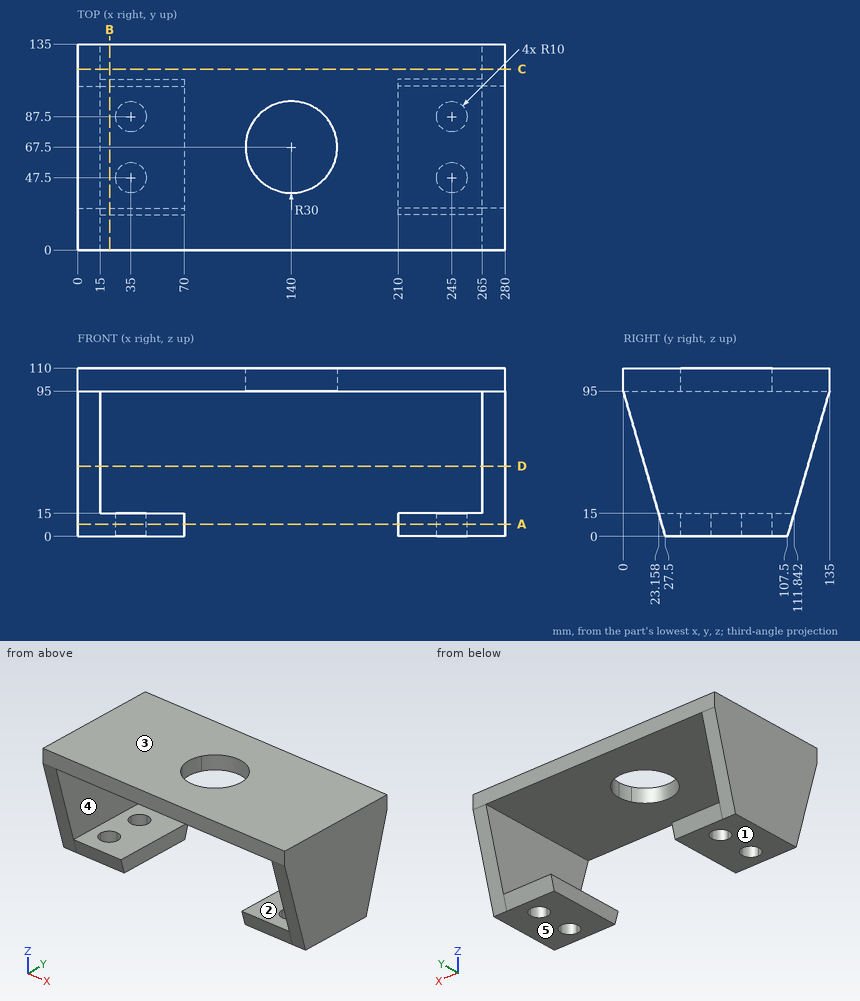
Can you work these out from the drawing? Everything is in mm from the part's minimum corner. A direction names the side the tool comes from. Round coordinates to 2 decimals unless told otherwise and drop trailing zeros. Write each loop counter-clockwise with the first axis right and the second up, starting at its lowest first coordinate (ties: lowest second). Pieces come first, ordered by that corner, then holes. Notation, with made-up numbers: (33.25, 79) - (48.25, 79) arc R21 cw to (48.25, 112) - close; hole circle Ø3 at (74.25, -0.5). An arc over 180 degrees is marked (long way). Write each question's results on one line, items separated by ' | '. Start each with the question number.
1) Please list where these lines run through material, in increasing order: line 1 (Z direction, x = 223, y = 82.5); line 2 (X direction, y = 30, z = 62.5); line 3 (Z direction, x = 82, y = 76.5).
2) Which directions (+Z, -Z, +X, -X, +Y, -Y) give clear straight access to the entire face, cutting with the end or side of a thin tool? Please do the marked faces 1 and 2.
3) Suppose I cut it at B-B (x = 21). List the corners of the cut face in (y, z) for me, and give its area (3 significant figures).
4) We'd pull the mould along Z, two halves only. Please class the marked faces 3, 4 and 5: released by +Z, released by -Z, zero draft, split by the parting line, or undercut.
5) Suppose I cut it at C-C (y = 118.5). List the corners of the cut face in (x, z) for me.
6) Suppose I cut it at D-D (z = 46). List the corners of the cut face in (x, y) for me.
7) Suppose I cut it at A-A (z = 8). List the corners of the cut face in (x, y) for me, and give its area (3 significant figures).
8) For pin 1 Ø6 at (x, z) = (216.5, 18.5) entering from -Y, with a flat end and sliding along its axis, tell me the tip position at first contact or that it passes through.
Here are the results:
1) line 1: z = 0 to 15, 95 to 110 | line 2: x = 0 to 15, 265 to 280 | line 3: z = 95 to 110
2) face 1: -Z, +X, -X, +Y, -Y | face 2: +Y, -Y
3) outline: (0, 95) - (135, 95) - (135, 110) - (0, 110) - close; (23.16, 15) - (27.5, 0) - (107.5, 0) - (111.84, 15) - close | area: 3,290 mm2
4) face 3: released by +Z | face 4: undercut | face 5: released by -Z
5) outline: (0, 38) - (15, 38) - (15, 95) - (265, 95) - (265, 38) - (280, 38) - (280, 110) - (0, 110) - close
6) outline: (0, 14.18) - (15, 14.18) - (15, 120.82) - (0, 120.82) - close; (265, 14.18) - (280, 14.18) - (280, 120.82) - (265, 120.82) - close
7) outline: (0, 25.18) - (70, 25.18) - (70, 109.82) - (0, 109.82) - close; (210, 25.18) - (280, 25.18) - (280, 109.82) - (210, 109.82) - close; hole circle Ø20 at (35, 47.5); hole circle Ø20 at (35, 87.5); hole circle Ø20 at (245, 47.5); hole circle Ø20 at (245, 87.5) | area: 10,600 mm2
8) pin 1: passes through
